Read the model definition and answer for the solid it produces. Units are mm, in the model's axes. Face numbers are marked on the shaded views. A direction names the side the tool comes from. Coordinates: 2 decimals unless noted, no trailing zeros. Order: outer loops, then holes, each group sorted by start corner. A loop starts at its lowest first (then second) coordinate and runs counter-clockwise, first axis right, second up. Notation, with made-up numbers: (8, 81.5) - (44, 81.5) arc R34 ccw to (44, 116.5) - close; hole circle Ø11 at (-18, 74.25). An arc over 180 degrees is marked (long way). Write item = value, one per line.
from build123d import *

# Parameters (mm, degrees)
SKETCH1_R           = 1.525
SKETCH1_W           = 3.5
SKETCH1_H           = 3.5
BOSS_EXTRUDE1_DEPTH = 3.5
FILLET1_R           = 2
FILLET2_R           = 2
FILLET3_R           = 5


with BuildPart() as part:
    # Sketch1 → Boss-Extrude1 (new body)
    with BuildSketch(Plane.XY):
        with BuildLine():
            Line((-11.8, 0), (11.8, 0))
            Line((11.8, 0), (11.8, 22.88))
            Line((11.8, 22.88), (3.175426481, 22.88))
            Line((3.175426481, 22.88), (9.058921367, 33.070512069))
            ThreePointArc((9.058921367, 33.070512069), (13.458683639, 38.149648334), (6.752404736, 38.575508076))
            Line((6.752404736, 38.575508076), (-2.309401077, 22.88))
            Line((-2.309401077, 22.88), (-11.8, 22.88))
            Line((-11.8, 22.88), (-11.8, 0))
        make_face()
        with Locations((0, 19.38)):
            Circle(SKETCH1_R, mode=Mode.SUBTRACT)
        with Locations((10, 36.700508076)):
            Circle(SKETCH1_R, mode=Mode.SUBTRACT)
        with Locations((-8.05, 3.75)):
            Rectangle(SKETCH1_W, SKETCH1_H, mode=Mode.SUBTRACT)
        with Locations((8.05, 3.75)):
            Rectangle(SKETCH1_W, SKETCH1_H, mode=Mode.SUBTRACT)
        with Locations((8.05, 13.63)):
            Rectangle(SKETCH1_W, SKETCH1_H, mode=Mode.SUBTRACT)
        with Locations((-8.05, 13.63)):
            Rectangle(SKETCH1_W, SKETCH1_H, mode=Mode.SUBTRACT)
    extrude(amount=BOSS_EXTRUDE1_DEPTH)

    # Fillet1
    fillet1_edges = [part.edges().sort_by_distance(p)[0] for p in [
        (-11.8, 22.88, 1.75),
        (11.8, 22.88, 1.75),
        (11.8, 0, 1.75),
        (-11.8, 0, 1.75),
    ]]
    fillet(fillet1_edges, radius=FILLET1_R)

    # Fillet2
    fillet2_edges = [part.edges().sort_by_distance(p)[0] for p in [
        (9.058921367, 33.070512069, 1.75),
        (3.175426481, 22.88, 1.75),
    ]]
    fillet(fillet2_edges, radius=FILLET2_R)

    # Fillet3
    fillet3_edges = [part.edges().sort_by_distance(p)[0] for p in [
        (-2.309401077, 22.88, 1.75),
    ]]
    fillet(fillet3_edges, radius=FILLET3_R)


solid = part.part
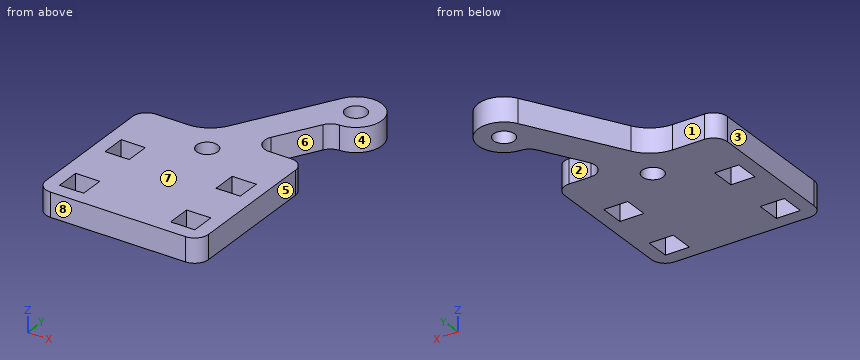
1) For the marked faces 1, 2, 3, 4 and 5, determine the directions among +Z, -Z, +X, -X, +Y, -Y from which every point of the face is accessible in a straight line to the end or side of a thin tool.
Returned:
face_1 = +Z, -Z, -X, +Y
face_2 = +Z, -Z, +X
face_3 = +Z, -Z, -X, +Y, -Y
face_4 = +Z, -Z
face_5 = +Z, -Z, +X, -Y
2) Straight lines are drawn through the part: line 1 along X through (y, z) = (13.5, 1.65); line 2 along Y through (x, z) = (10, 1.95); line 3 along Y through (x, z) = (-8.5, 0.9). For each, find the intervals that lie inside material, in ascending order. Write a range as from..to.
Returned:
line_1 = -11.8..-9.8, -6.3..6.3, 9.8..11.8
line_2 = 0.01..22.87, 32.95..35.18, 38.23..40.45
line_3 = 0..2, 5.5..11.88, 15.38..22.88
3) The part is cut by section A-A (y = 19.38). Determine the outline of the cut face in (x, z) (3 decimals), and give its area (3 significant figures).
Returned:
outline = (-11.8, 0) - (-1.525, 0) - (-1.525, 3.5) - (-11.8, 3.5) - close; (1.525, 0) - (11.8, 0) - (11.8, 3.5) - (1.525, 3.5) - close
area = 71.9 mm^2
4) Flat-ended cylindrical pins translate along their axes: pin 1 Ø1 at (y, z) = (13, 1) entering from +X; pin 2 Ø1 at (x, z) = (-7.5, 1.5) entering from +Y; pin 3 Ø1.6 at (x, z) = (8, 1.5) entering from +Y. Find the tip coordinate at first contact, or state that the pin passes through.
Returned:
pin_1 = 11.8
pin_2 = 22.88
pin_3 = 40.25
5) Determine the mould class of the marked faces 6, 7 and 8 for opening direction Y: pulls with the +Y half, pulls with the -Y half, needs draft (parallel to the pull), parting line crosses it, or undercut.
Returned:
face_6 = undercut
face_7 = needs draft
face_8 = pulls with the -Y half
6) The part is cut by section D-D (y = 7.5). Determine the outline of the cut face in (x, z), and give its area (3 significant figures).
Returned:
outline = (-11.8, 0) - (11.8, 0) - (11.8, 3.5) - (-11.8, 3.5) - close
area = 82.6 mm^2
7) The part is cut by section B-B (z = 0.95). Count the separate pieces of the cut face and the enclosed holes in it, and give its area (3 significant figures).
Returned:
separate_pieces = 1
enclosed_holes = 6
area = 586 mm^2
8) The part is cut by section C-C (x = 9). Determine the outline of the cut face in (y, z), and give its area (3 significant figures).
Returned:
outline = (0, 0) - (2, 0) - (2, 3.5) - (0, 3.5) - close; (5.5, 0) - (11.88, 0) - (11.88, 3.5) - (5.5, 3.5) - close; (15.38, 0) - (22.88, 0) - (22.88, 3.5) - (15.38, 3.5) - close; (32.59, 0) - (35.55, 0) - (35.55, 3.5) - (32.59, 3.5) - close; (37.85, 0) - (40.31, 0) - (40.31, 3.5) - (37.85, 3.5) - close
area = 74.6 mm^2
